Source: CAD feature listing. Evaluate the final solid. Frame: model axes, mm. A direction names the side the tool comes from. Round coordinates to 2 decimals unless told otherwise and drop trailing zeros. Loops run counter-clockwise (first coordinate to the right, second up) from the corner with the lowest first, then second, coordinate; pieces in that order, holes last. Notation, with made-up numbers: (48, -31) - (74, -31) arc R27 cw to (74, -1) - close; hole circle Ø1 at (55.5, 35.5). An arc over 180 degrees is marked (long way). Write item = value, one per line. Start each with the question number.
from build123d import *

# Parameters (mm, degrees)
F3_W        = 6.5772142261
F3_H        = 0.2320141066
F3_H_2      = 0.1190071926
F3_W_2      = 0.2564042807
F4_DEPTH    = 44.915836
F0_W        = 6.5772142261
F0_H        = 0.8592968807
F1_DEPTH    = 2.2352
F5_W        = 0.5953289354
F5_H        = 0.37034665
F6_DEPTH    = 0.03048
F7_T4_DEPTH = 1.9017438932
F2_SIZE     = 0.0254


# Not quite as in the source:
# - a fillet or chamfer that OpenCascade refuses, or shapes differently, is made with other operations: its cross-section is extruded or revolved along the edge and cut away or added


with BuildPart() as f4:
    # F3 (on Front) → F4 (new body)
    with BuildSketch(Plane.XZ):
        with Locations((0.5059395559, 0.0361560378)):
            Rectangle(F3_W, F3_H)
        with Locations((0.5059395559, 0.2116666874)):
            Rectangle(F3_W, F3_H_2)
        with Locations((0.5059395559, -0.1393546117)):
            Rectangle(F3_W, F3_H_2)
        with Locations((-2.9108696975, 0.0361560378)):
            Rectangle(F3_W_2, F3_H)
        with Locations((3.9227488093, 0.0361560378)):
            Rectangle(F3_W_2, F3_H)
    extrude(amount=F4_DEPTH)

    # F0 (on face) → F1 (join)
    with BuildSketch(Plane.XY.offset(0.2711702837)):
        with Locations((0.5059395559, -0.4296487314)):
            Rectangle(F0_W, F0_H)
    extrude(amount=F1_DEPTH)

    # F5 (on face) → F6 (join)
    with BuildSketch(Plane.XY.offset(2.5063702837)):
        with Locations((0.5059395559, -0.4296485859)):
            Rectangle(F5_W, F5_H)
    extrude(amount=F6_DEPTH)

    # F7: chamfer of 0.254 on 1 edges, made by hand


with BuildPart() as f7_tool2:
    # F7_s3 → F7_t4 (new body)
    with BuildSketch(Plane.YZ.offset(1.4568115025)):
        Polygon((-0.2444752608, 2.2828502837), (-0.4984752608, 2.5368502837), (-0.2444752608, 2.5368502837), align=None)
    extrude(amount=-F7_T4_DEPTH)

    split(bisect_by=Plane.XY.offset(2.5063702837), keep=Keep.TOP)


with BuildPart() as f4_1:
    add(f4.part)

    # F7_t1: cut F7_tool2
    add(f7_tool2.part, mode=Mode.SUBTRACT)

    # F2
    f2_edges = [f4_1.edges().sort_by_distance(p)[0] for p in [
        (0.50594, -0.614822, 2.53685),
    ]]
    chamfer(f2_edges, length=F2_SIZE)


solid = f4_1.part
(1) Cut plane A-A (y = -26). Output: boundary loops of the cut face in (x, z).
(2) Cut plane B-B (x = -1). Output: boundary loops of the cut face in (y, z), and give its area (3 significant figures).
(3) Pin query (flat end, axial travel): P1, Ø4, axis at x = 0, y = -32.5, coming from the +Z side. Return the tip coordinate at first contact, or that it passes through.
(4) Material intervals for line 1 along Y through (x, z) = (3.5, 0.35); line 2 along Z through (x, y) = (-2.5, -5); line 3 along X through (y, z) = (-7.5, 0.2), sorted ascending. Write a range as from..to.
(5) Cut plane C-C (z = 0.8). Output: boundary loops of the cut face in (x, y), and give its area (3 significant figures).
(6) Access query for faces 1 (the face through (0, -0.859, 1)), 2 (the face through (0, -22, -0.199)). Directions: +Z, -Z, +X, -X, +Y, -Y. A direction counts if a zero-diameter tool reaches every point of the face in a straight line with its end or side. Return the directions, or none.
Solution:
q1.outline = (-3.04, -0.08) - (-2.78, -0.08) - (-2.78, -0.2) - (3.79, -0.2) - (3.79, -0.08) - (4.05, -0.08) - (4.05, 0.15) - (3.79, 0.15) - (3.79, 0.27) - (-2.78, 0.27) - (-2.78, 0.15) - (-3.04, 0.15) - close
q2.outline = (-44.92, -0.2) - (0, -0.2) - (0, 2.51) - (-0.86, 2.51) - (-0.86, 0.27) - (-44.92, 0.27) - close
q2.area = 23.0 mm^2
q3.P1 = 0.27
q4.line_1 = -0.86..0
q4.line_2 = -0.2..0.27
q4.line_3 = -2.78..3.79
q5.outline = (-2.78, -0.86) - (3.79, -0.86) - (3.79, 0) - (-2.78, 0) - close
q5.area = 5.65 mm^2
q6.face_1 = +Z, +X, -X, -Y
q6.face_2 = -Z, +X, -X, +Y, -Y
